from build123d import *

# Parameters (mm, degrees)
SKETCH1_W           = 180
SKETCH1_H           = 180
BOSS_EXTRUDE1_DEPTH = 3
FILLET1_R           = 10
SKETCH2_R           = 1.7
CUT_EXTRUDE1_DEPTH  = 3
CUT_EXTRUDE2_DEPTH  = 128.314571044


with BuildPart() as part:
    # Sketch1 → Boss-Extrude1 (new body)
    with BuildSketch(Plane(origin=(0, 0, 0), x_dir=(1, 0, 0), z_dir=(0, 1, 0))):
        Rectangle(SKETCH1_W, SKETCH1_H)
    extrude(amount=BOSS_EXTRUDE1_DEPTH)

    # Fillet1
    fillet1_edges = [part.edges().sort_by_distance(p)[0] for p in [
        (90, 1.5, 90),
        (-90, 1.5, 90),
        (-90, 1.5, -90),
        (90, 1.5, -90),
    ]]
    fillet(fillet1_edges, radius=FILLET1_R)

    # Sketch2 → Cut-Extrude1 (cut)
    with BuildSketch(Plane(origin=(0, 3, 0), x_dir=(1, 0, 0), z_dir=(0, 1, 0))):
        with Locations(Location((-82, 75, 0), (0, 0, 270))):
            Circle(SKETCH2_R)
        with Locations(Location((-68, 75, 0), (0, 0, 270))):
            Circle(SKETCH2_R)
        with Locations(Location((68, 75, 0), (0, 0, 270))):
            Circle(SKETCH2_R)
        with Locations(Location((82, 75, 0), (0, 0, 270))):
            Circle(SKETCH2_R)
        with Locations(Location((-82, -75, 0), (0, 0, 270))):
            Circle(SKETCH2_R)
        with Locations(Location((-68, -75, 0), (0, 0, 270))):
            Circle(SKETCH2_R)
        with Locations(Location((68, -75, 0), (0, 0, 270))):
            Circle(SKETCH2_R)
        with Locations(Location((82, -75, 0), (0, 0, 270))):
            Circle(SKETCH2_R)
        with Locations(Location((-54, -75, 0), (0, 0, 270))):
            Circle(SKETCH2_R)
        with Locations(Location((54, -75, 0), (0, 0, 270))):
            Circle(SKETCH2_R)
        with Locations(Location((-40, -75, 0), (0, 0, 270))):
            Circle(SKETCH2_R)
        with Locations(Location((40, -75, 0), (0, 0, 270))):
            Circle(SKETCH2_R)
    extrude(amount=-CUT_EXTRUDE1_DEPTH, mode=Mode.SUBTRACT)

    # Sketch3 → Cut-Extrude2 (cut, through all)
    with BuildSketch(Plane(origin=(0, 3, 0), x_dir=(1, 0, 0), z_dir=(0, 1, 0))):
        with BuildLine():
            Line((-52, 40), (-52, -40))
            ThreePointArc((-52, -40), (-60, -48), (-68, -40))
            Line((-68, -40), (-68, 40))
            ThreePointArc((-68, 40), (-60, 48), (-52, 40))
        make_face()
        with BuildLine():
            Line((68, 40), (68, -40))
            ThreePointArc((68, -40), (60, -48), (52, -40))
            Line((52, -40), (52, 40))
            ThreePointArc((52, 40), (60, 48), (68, 40))
        make_face()
    extrude(amount=-CUT_EXTRUDE2_DEPTH, mode=Mode.SUBTRACT)


solid = part.part
For this review, take the finished solid that the model builds, in its own axes (mm). A direction names the side the tool comes from. Give positions to 0.01 mm unless a question says otherwise; leave off trailing zeros. Loops run counter-clockwise (first coordinate to the right, second up) from the corner with the lowest first, then second, coordinate; pieces in that order, holes last.
Item 1: Draft analysis for pull direction X (two halves, no side actions). For faces 1 (the cylindrical face through (60, 2, -48)), 2 (the cylindrical face through (87.15, 1.52, -86.99)), 3 (the flat face through (-1, 0, -1)), state which applies: +X half, -X half, draft (parallel to the pull), parting line (faces both ways), or undercut.
Item 2: For line 1 along X through (y, z) = (2.3, -15); line 2 along X through (y, z) = (0.65, -75); line 3 along Z through (x, y) = (-82, 0.8), list the stretches that pass through material, from the lowest coordinate up.
Item 3: Take a section at B-B, the plane y = 0.75. Give the number of separate pieces and of enclosed holes in the cut face, and give its area (3 significant figures).
Item 4: Tool access review of faces 4 (the cylindrical face through (-60, 2, -48)), 5 (the flat face through (-1, 3, -1)): name each direction out of +Z, -Z, +X, -X, +Y, -Y from which nothing blocks a thin tool from reaching the whole face with its end or side.
Item 5: Take a section at A-A, the plane z = 37. State the section outline as (x, y) points, and give its area (3 significant figures).
Calculated:
1. face 1: undercut
1. face 2: +X half
1. face 3: draft
2. line 1: x = -90 to -68, -52 to 52, 68 to 90
2. line 2: x = -90 to -83.7, -80.3 to -69.7, -66.3 to 66.3, 69.7 to 80.3, 83.7 to 90
2. line 3: z = -89.8 to -76.7, -73.3 to 73.3, 76.7 to 89.8
3. separate pieces: 1
3. enclosed holes: 14
3. area: 29,200 mm2
4. face 4: +Y, -Y
4. face 5: +Z, -Z, +X, -X, +Y
5. outline: (-90, 0) - (-68, 0) - (-68, 3) - (-90, 3) - close; (-52, 0) - (52, 0) - (52, 3) - (-52, 3) - close; (68, 0) - (90, 0) - (90, 3) - (68, 3) - close
5. area: 444 mm2
